Can you work these out from the model? Positions are in its coordinate system, mm. Face numbers are marked on the shaded views. A direction names the side the tool comes from. Give positions to 0.01 mm unless a question says otherwise; leave off trailing zeros. Order: outer loops, then holes, each group sorted by start corner. A loop starts at its lowest first (then second) coordinate and runs counter-clockwise, first axis right, second up. Notation, with made-up numbers: M -27.75,-16 L 28.25,-16 A24 ccw 28.25,2 Z; hole C 1.5,-11 d5. An arc over 180 degrees is marked long. Answer as a JSON object with one key per item and string values.
```python
from build123d import *
from build123d.topology import SkipClean

# Parameters (mm, degrees)
IZIM3_OUTSIDE_W             = 75.494
IZIM3_OUTSIDE_H             = 75.494
KES_EKSTR_ZYON1_DEPTH       = 7.5
IZIM4_R                     = 8.75
Y_KSEKLIK_EKSTR_ZYON1_DEPTH = 20
RADYUS1_R                   = 5
KES_EKSTR_ZYON2_DEPTH       = 20
IZIM6_R                     = 1.5
KES_EKSTR_ZYON3_DEPTH       = 60.476886267
IZIM7_R                     = 3.125
KES_EKSTR_ZYON4_DEPTH       = 11
KES_EKSTR_ZYON5_START       = -5
IZIM8_R                     = 8.75
KES_EKSTR_ZYON5_DEPTH       = 5
KES_EKSTR_ZYON6_DEPTH       = 2.5
IZIM11_R                    = 7.5


with BuildPart() as part:
    # Çizim1 → Döndür1 (revolve)
    with BuildSketch(Plane(origin=(0, 0, 0), x_dir=(1, 0, 0), z_dir=(0, 1, 0)), mode=Mode.PRIVATE) as d_nd_r1_sk:
        Polygon((-27.5, 25), (-27.5, 12), (-24.975, 12), (-24.975, -25), (0, -25), (0, 25), align=None)
    revolve(d_nd_r1_sk.sketch.rotate(Axis((0, 0, 25), (0, 0, -1)), 180), axis=Axis((0, 0, 25), (0, 0, -1)))

    # Çizim3 outside → Kes-Ekstrüzyon1 (cut)
    with BuildSketch(Plane(origin=(0, 0, -25), x_dir=(-1, 0, 0), z_dir=(0, 0, -1))):
        Rectangle(IZIM3_OUTSIDE_W, IZIM3_OUTSIDE_H)
        Polygon((15, 0), (7.5, 12.990381057), (-7.5, 12.990381057), (-15, 0), (-7.5, -12.990381057), (7.5, -12.990381057), align=None, mode=Mode.SUBTRACT)
    extrude(amount=-KES_EKSTR_ZYON1_DEPTH, mode=Mode.SUBTRACT)

    # Çizim4 → Yükseklik-Ekstrüzyon1 (add)
    with BuildSketch(Plane.XY.offset(25)):
        Circle(IZIM4_R)
    extrude(amount=Y_KSEKLIK_EKSTR_ZYON1_DEPTH)

    # Radyus1
    radyus1_edges = [part.edges().sort_by_distance(p)[0] for p in [
        (-8.75, 0, 25),
    ]]
    fillet(radyus1_edges, radius=RADYUS1_R)

    # Çizim5 → Kes-Ekstrüzyon2 (cut)
    with BuildSketch(Plane.XY.offset(45)):
        with BuildLine():
            Line((-2.291287847, 2.125), (2.291287847, 2.125))
            ThreePointArc((2.291287847, 2.125), (0, -3.125), (-2.291287847, 2.125))
        make_face()
    extrude(amount=-KES_EKSTR_ZYON2_DEPTH, mode=Mode.SUBTRACT)

    # Çizim6 → Kes-Ekstrüzyon3 (cut, through all)
    with BuildSketch(Plane(origin=(0, 0, 0), x_dir=(1, 0, 0), z_dir=(0, 1, 0))):
        with Locations(Location((0, -35.5, 0), (0, 0, 90))):
            Circle(IZIM6_R)
    extrude(amount=KES_EKSTR_ZYON3_DEPTH, mode=Mode.SUBTRACT)

    # Çizim7 → Kes-Ekstrüzyon4 (cut)
    with SkipClean():  # the faces are left unmerged after this step: merging them gives an invalid solid
        with BuildSketch(Plane.XY.offset(45)):
            Circle(IZIM7_R)
        extrude(amount=-KES_EKSTR_ZYON4_DEPTH, mode=Mode.SUBTRACT)

    # Çizim8 → Kes-Ekstrüzyon5 (cut)
    with SkipClean():  # the faces are left unmerged after this step: merging them gives an invalid solid
        with BuildSketch(Plane.XY.offset(45).offset(KES_EKSTR_ZYON5_START)):
            with Locations(Location((0, 0, 0), (0, 0, 180))):
                Circle(IZIM8_R)
        extrude(amount=KES_EKSTR_ZYON5_DEPTH, mode=Mode.SUBTRACT)

    # Çizim9 → Kes-Ekstrüzyon6 (cut)
    with SkipClean():  # the faces are left unmerged after this step: merging them gives an invalid solid
        with BuildSketch(Plane(origin=(0, 0, -25), x_dir=(-1, 0, 0), z_dir=(0, 0, -1))):
            Polygon((7.5, -12.990381057), (15, 0), (7.5, 12.990381057), (-7.5, 12.990381057), (-15, 0), (-7.5, -12.990381057), align=None)
        extrude(amount=-KES_EKSTR_ZYON6_DEPTH, mode=Mode.SUBTRACT)

    # Kes-Süpür1: sweep along a path in Çizim10
    with SkipClean():  # the faces are left unmerged after this step: merging them gives an invalid solid
        with BuildLine(Plane(origin=(0, 0, 0), x_dir=(1, 0, 0), z_dir=(0, 1, 0))) as kes_s_p_r1_path:
            Line((0, 22.5), (0, 0))
            Line((0, 0), (-24.975, -25))
        # Çizim11 → Kes-Süpür1 (sweep, cut)
        with BuildSketch(Plane(origin=(0, 0, -22.5), x_dir=(-1, 0, 0), z_dir=(0, 0, -1))):
            Circle(IZIM11_R)
        sweep(path=kes_s_p_r1_path.line, transition=Transition.RIGHT, mode=Mode.SUBTRACT)


solid = part.part
```
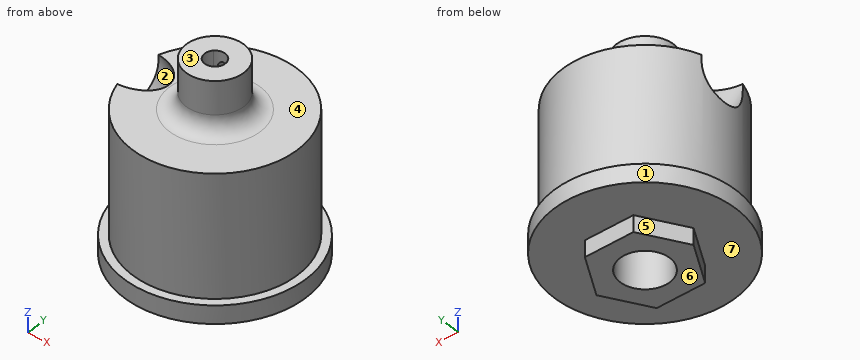
1) I want a section at C-C on y = 19.5. Write out the boundary of the cut face in (x, z), and give its area (3 significant figures).
Results found:
{"outline": "M -19.39,-17.5 L 19.39,-17.5 L 19.39,-12 L 15.6,-12 L 15.6,25 L -15.6,25 L -15.6,-12 L -19.39,-12 Z", "area": "1,370 mm²"}
2) I want a section at A-A on z = 31. Write out the boundary of the cut face in (x, y) (3 decimals).
Results found:
{"outline": "C 0,0 d17.5; hole M -2.291,2.125 A3.125 ccw long 2.291,2.125 Z"}
3) I want a section at B-B on y = -22.5. Write out the boundary of the cut face in (x, z).
Results found:
{"outline": "M -15.81,-17.5 L 15.81,-17.5 L 15.81,-12 L 10.84,-12 L 10.84,25 L -10.84,25 L -10.84,-12 L -15.81,-12 Z"}
4) I need wall thicknesses on L1, parallel to Y at x = 0, z = -7 (3 decimals); L2, parallel to Y at x = 0, z = 32.75 (3 decimals); L3, parallel to X at y = 0, z = 33 (3 decimals). Which ranges of each line are inside material? Lowest first, please.
Results found:
{"L1": "y = -24.975 to -7.5, 7.5 to 24.975", "L2": "y = -8.75 to -3.125, 2.125 to 8.75", "L3": "x = -8.75 to -3.125, 3.125 to 8.75"}
5) Thinking about a two-plate mould opening in X: for the marked faces 1, 2 and 3, which applies, pulls with the +X half, pulls with the -X half, needs draft (parallel to the pull), parting line crosses it, or undercut?
Results found:
{"face 1": "parting line crosses it", "face 2": "undercut", "face 3": "needs draft"}
6) I'm going to push flat-ended pins straight in: pin 1 Ø1.6 at (x, y) = (0.5, -0.5) entering from +Z; pin 2 Ø2 at (y, z) = (0, 14) entering from +X (3 decimals); pin 3 Ø5 at (x, z) = (-0.5, 28.5) entering from -Y. Where does each tip first touch, or does it pass through?
Results found:
{"pin 1": "stops at z = 25", "pin 2": "stops at x = 24.975", "pin 3": "stops at y = -10.74"}
7) For the marked faces 4, 5, 6 and 7, which set-ups out of +Z, -Z, +X, -X, +Y, -Y let a thin tool reach every point of the face, with its end or its side?
Results found:
{"face 4": "+Z", "face 5": "-Z, -X, +Y", "face 6": "-Z, +X, -X, +Y, -Y", "face 7": "-Z"}
